```python
from build123d import *

# Parameters (mm, degrees)
F1_DEPTH = 48.26
F2_R     = 75.1298165033
F3_DEPTH = 4.064
F6_DEPTH = 1.524
F7_DEPTH = 1.524
F9_DEPTH = 196.088


with BuildPart() as f1:
    # F0 (on Front) → F1 (new body)
    with BuildSketch(Plane.XZ):
        with BuildLine():
            ThreePointArc((-34.4267364961, -67.788390466), (39.7682207439, -64.7993417143), (76.0293763472, 0))
            ThreePointArc((76.0293763472, 0), (76.0019863824, 2.0406209035), (75.9198362228, 4.0797715191))
            ThreePointArc((75.9198362228, 4.0797715191), (34.4267338783, 67.7883917955), (-41.4931009863, 63.7086229507))
            ThreePointArc((-41.4931009863, 63.7086229507), (-75.9198364409, -4.0797674593), (-34.4267364961, -67.788390466))
        make_face()
        with BuildLine():
            Line((-151.8396729123, -8.159534353), (-34.4267364961, -67.788390466))
            ThreePointArc((-34.4267364961, -67.788390466), (-75.9198364409, -4.0797674593), (-41.4931009863, 63.7086229507))
            Line((-41.4931009863, 63.7086229507), (-151.8396729123, -8.159534353))
        make_face()
        with BuildLine():
            ThreePointArc((-41.4931009863, 63.7086229507), (34.4267338783, 67.7883917955), (75.9198362228, 4.0797715191))
            Line((75.9198362228, 4.0797715191), (68.8534724234, 135.5767812208))
            Line((68.8534724234, 135.5767812208), (-41.4931009863, 63.7086229507))
        make_face()
        with BuildLine():
            ThreePointArc((75.9198362228, 4.0797715191), (76.0019863824, 2.0406209035), (76.0293763472, 0))
            ThreePointArc((76.0293763472, 0), (39.7682207439, -64.7993417143), (-34.4267364961, -67.788390466))
            Line((-34.4267364961, -67.788390466), (82.9862004889, -127.4172468679))
            Line((82.9862004889, -127.4172468679), (75.9198362228, 4.0797715191))
        make_face()
    extrude(amount=F1_DEPTH)

    # F2 (on face) → F3 (join)
    with BuildSketch(Plane(origin=(0, 0, 0), x_dir=(-1, 0, 0), z_dir=(0, 1, 0))):
        Circle(F2_R)
    extrude(amount=F3_DEPTH)

    # F4 (on face) + F5 (on face) → F6 (join)
    with BuildSketch(Plane(origin=(0, 4.064, 0), x_dir=(-1, 0, 0), z_dir=(0, 1, 0))):
        Polygon((21.1120117456, -12.1532529593), (36.5837341302, 65.6210311174), (-22.6685176048, 16.9392599994), (-37.0748307403, -65.3448257584), align=None)
    with BuildSketch(Plane(origin=(0, 4.064, 0), x_dir=(-1, 0, 0), z_dir=(0, 1, 0))):
        Polygon((-11.7188123986, -16.5306981653), (21.1120117456, -11.42368), (12.0517571455, 16.7637839913), (-23.2249982655, 16.7637839913), align=None)
    extrude(amount=F6_DEPTH)

    # F5 (on face) + F6_face (on face) → F7 (join)
    with BuildSketch(Plane(origin=(0, 4.064, 0), x_dir=(-1, 0, 0), z_dir=(0, 1, 0))):
        Polygon((-11.7188123986, -16.5306981653), (21.1120117456, -11.42368), (12.0517571455, 16.7637839913), (-23.2249982655, 16.7637839913), align=None)
    with BuildSketch(Plane(origin=(0.8615921518, 5.588, 1.1811459069), x_dir=(-1, 0, 0), z_dir=(0, 1, 0))):
        Polygon((-36.2132385885, -66.5259716654), (21.9736038974, -13.3343988662), (37.445326282, 64.4398852105), (-21.806925453, 15.7581140924), (-21.8376478253, 15.5826380844), (-22.3634061137, 15.5826380844), (-22.0144394867, 14.5728627107), align=None)
    extrude(amount=F7_DEPTH)

    # F8 (on face) → F9 (join)
    with BuildSketch(Plane.XZ.offset(48.26)):
        Polygon((-72.4382175174, 43.5542269979), (-72.4382175174, -48.4840343904), (-41.4931002444, -48.503398313), (-41.4931002444, -8.159534353), (0, -8.159534353), (0, 11.7922946811), (-41.4931002444, 11.7922946811), (-41.4931002444, 43.5542269979), align=None)
    extrude(amount=F9_DEPTH)


solid = f1.part
```
The model under review builds one solid part; all positions refer to its coordinate system, in mm. A direction names the side the tool comes from. Round coordinates to 2 decimals unless told otherwise and drop trailing zeros. Order: outer loops, then holes, each group sorted by start corner. A loop starts at its lowest first (then second) coordinate and runs counter-clockwise, first axis right, second up. Notation, with made-up numbers: (67.5, -18.5) - (109.5, -18.5) arc R29 ccw to (109.5, 5.5) - close; hole circle Ø2 at (77, 9). An arc over 180 degrees is marked (long way). Answer in a Markdown table with one row per item.
(1) Machinability: for faces 1 (the face through (-20, -145, 11.792)), 2 (the face through (-95, -48.26, -2)), 3 (the face through (16.287, 2.004, -73.343)), 4 (the face through (8.39, 5.57, -39.12)), which of the approach directions +Z, -Z, +X, -X, +Y, -Y give a long, thin tool a straight path to every point of the face, cutting with its end or side? Answer none if there is none.
Result set:
| item | result |
|---|---|
| face 1 | +Z, +X, -Y |
| face 2 | +Z, -Z, -X, -Y |
| face 3 | +Y |
| face 4 | -Z, -X, +Y |
(2) Take a section at D-D on x = 63. Write out the cut boundary in (y, z), plus the area to 3 significant figures.
Result set:
| item | result |
|---|---|
| outline | (-48.26, -117.27) - (0, -117.27) - (0, -40.93) - (4.06, -40.93) - (4.06, 40.93) - (0, 40.93) - (0, 131.76) - (-48.26, 131.76) - close |
| area | 12,400 mm2 |
(3) Take a section at B-B on x = -31. Write out the cut boundary in (y, z), plus the area to 3 significant figures.
Result set:
| item | result |
|---|---|
| outline | (-244.35, -8.16) - (-48.26, -8.16) - (-48.26, -69.53) - (0, -69.53) - (0, -68.44) - (4.06, -68.44) - (4.06, 37.55) - (7.11, 37.55) - (7.11, 61.03) - (4.06, 61.03) - (4.06, 68.44) - (0, 68.44) - (0, 70.54) - (-48.26, 70.54) - (-48.26, 11.79) - (-244.35, 11.79) - close |
| area | 11,300 mm2 |
(4) Take a section at A-A on y = -160. Write out the cut boundary in (x, z), plus the area to 3 significant figures.
Result set:
| item | result |
|---|---|
| outline | (-72.44, -48.48) - (-41.49, -48.5) - (-41.49, -8.16) - (0, -8.16) - (0, 11.79) - (-41.49, 11.79) - (-41.49, 43.55) - (-72.44, 43.55) - close |
| area | 3,680 mm2 |
(5) Clearance check with flat-ended pins moving along their axes: P1, Ø1.5, axis at y = -196.5, z = -14.5, coming from the -X side; P2, Ø6, axis at y = -177, z = 1.5, coming from the +X side; P3, Ø1.5, axis at y = -42, z = 104, coming from the -X side. State where each tip first meets the part, or that it passes through.
Result set:
| item | result |
|---|---|
| P1 | stops at x = -72.44 |
| P2 | stops at x = 0 |
| P3 | stops at x = 19.22 |
(6) For line 1 (X direction, y = -103, z = 40.5); line 2 (Y direction, x = 72, z = -112.5); line 3 (Y direction, x = 28.5, z = -52.5), list the stretches that pass through material, from the lowest coordinate up. Write a range as from..to.
Result set:
| item | result |
|---|---|
| line 1 | x = -72.44..-41.49 |
| line 2 | y = -48.26..0 |
| line 3 | y = -48.26..7.11 |
(7) Take a section at C-C on z = 0. Write out the cut boundary in (x, y), plus the area to 3 significant figures.
Result set:
| item | result |
|---|---|
| outline | (-139.31, -48.26) - (-72.44, -48.26) - (-72.44, -244.35) - (0, -244.35) - (0, -48.26) - (76.14, -48.26) - (76.14, 0) - (75.13, 0) - (75.13, 4.06) - (25.63, 4.06) - (25.63, 7.11) - (-23.53, 7.11) - (-23.53, 4.06) - (-75.13, 4.06) - (-75.13, 0) - (-139.31, 0) - close |
| area | 25,400 mm2 |
